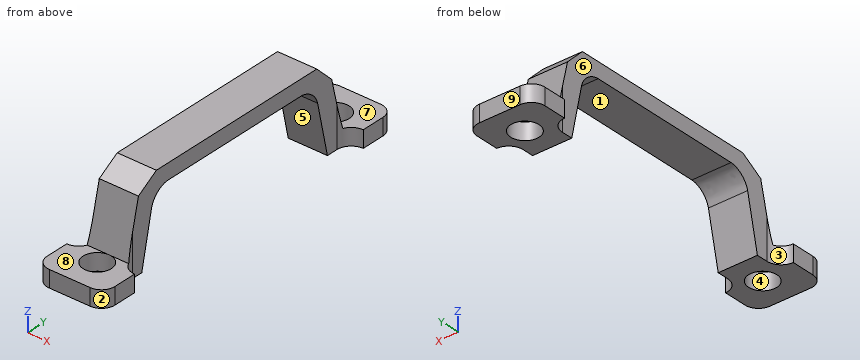
```python
from build123d import *
from OCP.BRepFilletAPI import BRepFilletAPI_MakeChamfer

# Parameters (mm, degrees)
SKETCH_1_W               = 10.068208361
SKETCH_1_H               = 51.310344827
SKETCH_1_R               = 2.1
EXTRUDE_1_DEPTH          = 2.5
EXTRUDE_2_REACH          = 83.327
CUT_EXTRUDE_1_DEPTH      = 83.243670079
CUT_EXTRUDE_1_DEPTH_BACK = 83.243670079
CUT_EXTRUDE_2_DEPTH      = 122.121367623
CUT_EXTRUDE_2_DEPTH_BACK = 122.121367623
FILLET_2_R               = 2
CHAMFER_2_SIZE           = 2
CHAMFER_2_SIZE2          = 2.70532723


with BuildPart() as part:
    # 草图1 → 凸台-拉伸1 (new body)
    with BuildSketch(Plane.XY):
        with Locations((84.451834639, -55.007101597)):
            Rectangle(SKETCH_1_W, SKETCH_1_H)
        with Locations((84.623869854, -34.007101596)):
            Circle(SKETCH_1_R, mode=Mode.SUBTRACT)
        with Locations((84.623869854, -76.007101596)):
            Circle(SKETCH_1_R, mode=Mode.SUBTRACT)
    extrude(amount=EXTRUDE_1_DEPTH)

    # 凸台-拉伸2: up to this face of the body (flat: up to its plane)
    extrude_2_end = Plane(part.part.faces().sort_by_distance((79.417730458, -55.007101596, 1.25))[0])
    # 草图2 → 凸台-拉伸2 (add, up to the picked face)
    with BuildSketch(Plane(origin=(89.485938819, 0, 0), x_dir=(0, 0, -1), z_dir=(1, 0, 0)), mode=Mode.PRIVATE) as extrude_2_sk1:
        Polygon((-12.5, -71.517171054), (-2.5, -73.914822505), (-2.5, -36.099380688), (-12.5, -38.497032139), align=None)
    extrude_2_tool1 = split(extrude(extrude_2_sk1.sketch, amount=-EXTRUDE_2_REACH, mode=Mode.PRIVATE), bisect_by=extrude_2_end, keep=Keep.BOTH, mode=Mode.PRIVATE)
    add(extrude_2_tool1.solids().sort_by(Axis((89.485939, -55.007102, 7.387173), (-1, 0, 0)))[0])

    # 草图3 → 切除-拉伸1 (cut, two sides: drawn at the far end of the back side and taken through both)
    with BuildSketch(Plane(origin=(89.485938819, 0, 0), x_dir=(0, 0, -1), z_dir=(1, 0, 0)).offset(-CUT_EXTRUDE_1_DEPTH_BACK)):
        Polygon((-10.198786391, -69.151033694), (0, -71.395312685), (0, -38.618890508), (-10.198786391, -40.863169498), align=None)
    extrude(amount=CUT_EXTRUDE_1_DEPTH + CUT_EXTRUDE_1_DEPTH_BACK, mode=Mode.SUBTRACT)

    # 草图4 → 切除-拉伸2 (cut, two sides: drawn at the far end of the back side and taken through both)
    with BuildSketch(Plane.XY.offset(12.5).offset(-CUT_EXTRUDE_2_DEPTH_BACK)):
        with BuildLine():
            Line((81.544440974, -36.941486908), (81.544440974, -73.072716285))
            ThreePointArc((81.544440974, -73.072716285), (79.417730458, -75.199426802), (77.291019941, -73.072716285))
            Line((77.291019941, -73.072716285), (77.291019941, -36.941486908))
            ThreePointArc((77.291019941, -36.941486908), (79.417730458, -34.814776391), (81.544440974, -36.941486908))
        make_face()
        with BuildLine():
            Line((87.359228302, -36.941486908), (87.359228302, -73.072716285))
            ThreePointArc((87.359228302, -73.072716285), (89.485938819, -75.199426802), (91.612649336, -73.072716285))
            Line((91.612649336, -73.072716285), (91.612649336, -36.941486908))
            ThreePointArc((91.612649336, -36.941486908), (89.485938819, -34.814776391), (87.359228302, -36.941486908))
        make_face()
    extrude(amount=CUT_EXTRUDE_2_DEPTH + CUT_EXTRUDE_2_DEPTH_BACK, mode=Mode.SUBTRACT)

    # 圆角1
    # a fillet whose section is not a circle: 3 mm, written as the material it adds along each edge
    with BuildSketch(Plane(origin=(87.359228302, -40.863169498, 10.198786391), x_dir=(0, 0.2149116520268582, -0.9766334941128564), z_dir=(-1, 0, 0)), Plane(origin=(87.359228302, -69.151033694, 10.198786391), x_dir=(0, 1, 0), z_dir=(-1, 0, 0))) as fillet_1_piece_1:
        with BuildLine():
            Bezier((2.411616085, 0), (0, 0), (-0.518284397, 2.355265044), weights=[1, 0.666666667, 1])
            Line((-0.518284397, 2.355265044), (0, 0))
            Line((0, 0), (2.411616085, 0))
        make_face()
    extrude(amount=5.814787328)

    # 圆角2
    fillet_2_edges = [part.edges().sort_by_distance(p)[0] for p in [
        (89.485938819, -80.66227401, 1.25),
        (79.417730458, -80.66227401, 1.25),
        (79.417730458, -29.351929183, 1.25),
        (89.485938819, -29.351929183, 1.25),
    ]]
    fillet(fillet_2_edges, radius=FILLET_2_R)

    # 倒角2: one chamfer whose edges measure the first distance from different faces: ONE call of the kernel's chamfer builder (chamfer() names one face for all edges)
    chamfer_2_edges_1 = [part.edges().sort_by_distance(p)[0] for p in [
        (84.451834638, -71.517171054, 12.5),
    ]]
    chamfer_2_side_1 = [part.faces().sort_by_distance(p)[0] for p in [
        (84.451834638, -72.722762821, 7.471780545),
    ]]
    chamfer_2_edges_2 = [part.edges().sort_by_distance(p)[0] for p in [
        (84.451834638, -38.497032139, 12.5),
    ]]
    chamfer_2_side_2 = [part.faces().sort_by_distance(p)[0] for p in [
        (84.451834638, -55.007101596, 12.5),
    ]]
    chamfer_2 = BRepFilletAPI_MakeChamfer(part.part.solid().wrapped)
    for e in chamfer_2_edges_1:
        chamfer_2.Add(CHAMFER_2_SIZE, CHAMFER_2_SIZE2, e.wrapped, chamfer_2_side_1[0].wrapped)  # the first distance lies on this face
    for e in chamfer_2_edges_2:
        chamfer_2.Add(CHAMFER_2_SIZE, CHAMFER_2_SIZE2, e.wrapped, chamfer_2_side_2[0].wrapped)  # the first distance lies on this face
    add(Compound.cast(chamfer_2.Shape()), mode=Mode.REPLACE)


solid = part.part
```
For this review, take the finished solid that the model builds, in its own axes (mm). Face numbers are marked on the shaded views. A direction names the side the tool comes from. Round coordinates to 2 decimals unless told otherwise and drop trailing zeros. Loops run counter-clockwise (first coordinate to the right, second up) from the corner with the lowest first, then second, coordinate; pieces in that order, holes last.
Q1. Add section C-C on y = -32.5. Write out the cut boundary in (x, z), plus the area to 3 significant figures.
Result sheet:
outline: (79.42, 0) - (83.16, 0) - (83.16, 2.5) - (79.42, 2.5) - close; (86.09, 0) - (89.49, 0) - (89.49, 2.5) - (86.09, 2.5) - close
area: 17.9 mm2
Q2. Add section A-A on z = 2. Write out the cut boundary in (x, y).
Result sheet:
outline: (79.42, -78.66) arc R2 ccw to (81.42, -80.66) - (87.49, -80.66) arc R2 ccw to (89.49, -78.66) - (89.49, -75.2) arc R2.13 cw to (87.36, -73.07) - (87.36, -70.96) - (81.54, -70.96) - (81.54, -73.07) arc R2.13 cw to (79.42, -75.2) - close; (79.42, -34.81) arc R2.13 cw to (81.54, -36.94) - (81.54, -39.06) - (87.36, -39.06) - (87.36, -36.94) arc R2.13 cw to (89.49, -34.81) - (89.49, -31.35) arc R2 ccw to (87.49, -29.35) - (81.42, -29.35) arc R2 ccw to (79.42, -31.35) - close; hole circle Ø4.2 at (84.62, -76.01); hole circle Ø4.2 at (84.62, -34.01)
Q3. Add section D-D on z = 4. Write out the cut boundary in (x, y), plus the area to 3 significant figures.
Result sheet:
outline: (81.49, -73.56) - (87.41, -73.56) arc R2.13 cw to (87.36, -73.07) - (87.36, -70.52) - (81.54, -70.52) - (81.54, -73.07) arc R2.13 cw to start; (81.49, -36.46) arc R2.13 cw to (81.54, -36.94) - (81.54, -39.5) - (87.36, -39.5) - (87.36, -36.94) arc R2.13 cw to (87.41, -36.46) - close
area: 35.4 mm2
Q4. Insertion check: pin 1 Ø3.5 at (x, y) = (84.62, -76.01) entering from -Z; pin 2 Ø2 at (x, z) = (84.5, 4) entering from +Y; pin 3 Ø1 at (x, z) = (84, 9.5) entering from +Y; pin 4 Ø2 at (x, y) = (86, -34) entering from +Z. Each pin has a flat end and moves straight along its axis. Give the tip position at first contact, or say it passes through.
Result sheet:
pin 1: passes through
pin 2: stops at y = -36.22
pin 3: stops at y = -37.66
pin 4: stops at z = 2.5
Q5. To check wall thickness, follow line 1 along Z through (x, y) = (87.75, -34.5); line 2 along Y through (x, z) = (87, 2.75); line 3 along Y through (x, z) = (86.5, 5.5). State the ranges of each line that lie inside material, in increasing order.
Result sheet:
line 1: z = 0 to 2.5
line 2: y = -73.85 to -70.79, -39.22 to -36.16
line 3: y = -73.2 to -70.19, -39.83 to -36.82
Q6. Machinability: for the marked faces 5, 6, 7, 8 and 9, which of the approach directions +Z, -Z, +X, -X, +Y, -Y give a long, thin tool a straight path to every point of the face, cutting with its end or side? Answer none if there is none.
Result sheet:
face 5: -Z, +X, -X
face 6: +Z, -Z, -X
face 7: +Z, +X, -X, +Y
face 8: +Z, +X, -X, -Y
face 9: +Z, -Z, +X, -X, +Y
Q7. Mouldability with a two-part tool opening along X and no side actions: class the marked faces 1, 2, 3 and 4 as +X half, -X half, draft (parallel to the pull), parting line (faces both ways), or undercut.
Result sheet:
face 1: draft
face 2: +X half
face 3: -X half
face 4: undercut
Q8. Add section B-B on x = 80.75. Write out the cut boundary in (y, z).
Result sheet:
outline: (-80.55, 0) - (-74.73, 0) - (-74.73, 2.5) - (-80.55, 2.5) - close; (-35.28, 0) - (-29.47, 0) - (-29.47, 2.5) - (-35.28, 2.5) - close
